from build123d import *

# Parameters (mm, degrees)
F1_DEPTH = 34
F2_W     = 4
F2_H     = 38
F2_W_2   = 21
F3_DEPTH = 50
F4_R     = 1.5
F5_R     = 0.5


with BuildPart() as f1:
    # F0 (on Top) → F1 (new body, symmetric)
    with BuildSketch(Plane.XY):
        Polygon((-1.5, 4), (-1.5, 0), (0, 0), (0, 5.5), (-10, 5.5), (-10, 35.5), (-11.5, 35.5), (-11.5, 4), align=None)
    extrude(amount=F1_DEPTH, both=True)

    # F2 (on face) → F3 (cut)
    with BuildSketch(Plane(origin=(-11.5, 0, 0), x_dir=(0, -1, 0), z_dir=(-1, 0, 0))):
        with Locations((-2, 0)):
            Rectangle(F2_W, F2_H)
        with Locations((-14.5, 0)):
            Rectangle(F2_W_2, F2_H)
    extrude(amount=-F3_DEPTH, mode=Mode.SUBTRACT)

    # F4
    f4_edges = [f1.edges().sort_by_distance(p)[0] for p in [
        (0, 5.5, -26.5),
        (0, 5.5, 26.5),
        (-11.5, 4, -26.5),
        (-11.5, 4, 26.5),
    ]]
    fillet(f4_edges, radius=F4_R)

    # F5
    f5_edges = [f1.edges().sort_by_distance(p)[0] for p in [
        (-10, 5.5, -26.5),
        (-10, 5.5, 26.5),
        (-1.5, 4, -26.5),
        (-1.5, 4, 26.5),
    ]]
    fillet(f5_edges, radius=F5_R)


solid = f1.part
Work out the finished part from the listing and answer in its coordinate system (mm). A direction names the side the tool comes from. Round coordinates to 2 decimals unless told otherwise and drop trailing zeros. Write each loop counter-clockwise with the first axis right and the second up, starting at its lowest first coordinate (ties: lowest second). Pieces come first, ordered by that corner, then holes. Notation, with made-up numbers: (87.5, -18.5) -> (121.5, -18.5) arc R15 ccw to (121.5, -10.5) -> close; hole circle Ø3 at (58.5, 89). An arc over 180 degrees is marked (long way). Answer as CSV lines item,"result". Start each with the question number.
(1) The part is cut by section C-C, the plane z = -20. Give the vertices of the cut face in (x, y).
(2) The part is cut by section D-D, the plane y = 30. Give the vertices of the cut face in (x, z).
(3) Each of these flat-tipped pins is pushed along its axis until it touches: pin 1 (1.6 mm diameter, centred on x = -10.5, z = -8, fed in from -Y); pin 2 (3 mm diameter, centred on y = 15.5, z = 21, fed in from +X); pin 3 (4 mm diameter, centred on x = -6.5, z = -29, fed in from -Y). Where does it stop, or does it pass through?
(4) The part is cut by section A-A, the plane y = 20.5. Give the vertices of the cut face in (x, z), then the cut area to 3 significant figures.
(5) The mould has two halves that part along Z. Classify faces 1 (the flat face through (-10.5, 16.5, 34)), 2 (the flat face through (0, 2, -26)), 3 (the flat face through (-11, 25, 0)): +Z half, -Z half, draft (parallel to the pull), parting line (faces both ways), or undercut.
(6) Find the intervals of material crossed by probe 1 along Z at (x, y) = (-10.5, 5); probe 2 along X at (y, z) = (32, 26); probe 3 along Y at (x, z) = (-7.75, -31), in increasing order.
(7) A tool of negligible diameter and unlimited length cuts with its end or side. For faces 4 (the flat face through (-6, 4, -26)), 5 (the flat face through (-10.5, 9.7, 19)), 6 (the flat face through (-11.5, 27, 0)), 7 (the flat face through (-5, 5.5, 27)), from which of +Z, -Z, +X, -X, +Y, -Y can it reach the whole face along a straight path? Write none if from no direction.
(8) The part is cut by section B-B, the plane x = -8.25. Give the vertices of the cut face in (y, z), then the cut area to 3 significant figures.
Output values:
1,outline,"(-11.5, 5.5) arc R1.5 ccw to (-10, 4) -> (-2, 4) arc R0.5 cw to (-1.5, 3.5) -> (-1.5, 0) -> (0, 0) -> (0, 4) arc R1.5 ccw to (-1.5, 5.5) -> (-9.5, 5.5) arc R0.5 cw to (-10, 6) -> (-10, 35.5) -> (-11.5, 35.5) -> close"
2,outline,"(-11.5, -34) -> (-10, -34) -> (-10, 34) -> (-11.5, 34) -> close"
3,pin 1,"stops at y = 25"
3,pin 2,"stops at x = -10"
3,pin 3,"stops at y = 4"
4,outline,"(-11.5, -34) -> (-10, -34) -> (-10, -19) -> (-11.5, -19) -> close; (-11.5, 19) -> (-10, 19) -> (-10, 34) -> (-11.5, 34) -> close"
4,area,"45.0 mm²"
5,face 1,"+Z half"
5,face 2,"draft"
5,face 3,"undercut"
6,probe 1,"z = -34 to -19, 19 to 34"
6,probe 2,"x = -11.5 to -10"
6,probe 3,"y = 4 to 5.5"
7,face 4,"+Z, -Z, -X, -Y"
7,face 5,"+X, -X, -Y"
7,face 6,"+Z, -Z, -X, +Y, -Y"
7,face 7,"+Z, -Z, +X, +Y"
8,outline,"(4, -34) -> (5.5, -34) -> (5.5, -19) -> (4, -19) -> close; (4, 19) -> (5.5, 19) -> (5.5, 34) -> (4, 34) -> close"
8,area,"45.0 mm²"
